Source: CAD feature listing. Evaluate the final solid. Frame: model axes, mm. A direction names the side the tool comes from. Round coordinates to 2 decimals unless told otherwise and drop trailing zeros. Order: outer loops, then holes, each group sorted by start corner. A loop starts at its lowest first (then second) coordinate and runs counter-clockwise, first axis right, second up. Notation, with made-up numbers: (46, 61.25) -> (64, 61.25) arc R26 ccw to (64, 80.25) -> close; hole circle Ø4 at (36.5, 33.5). An arc over 180 degrees is marked (long way). Write item = value, one per line. Start each with the question number.
(1) Cut plane A-A on y = -45. Return the cut outline in (x, z), then the cut area to 3 significant figures.
(2) Ray query, line 1 (Y direction, x = -73.5, z = 3.75); line 2 (X direction, y = -43.5, z = 10.5). Return the intervals inside material, ascending.
(3) Reachability of faces 1 (the face through (-82.914, -19, 9)), 2 (the face through (-63.864, -47, 9)) from +Z, -Z, +X, -X, +Y, -Y: full face, straight path, thin tool, end or side. Return the list, or none.
(4) Cut plane B-B on z = 16.75. Return the cut outline in (x, y), then the cut area to 3 significant figures.
(5) Contact query for flat-ended pins moving along their axis: pin 1 Ø5.5 at (y, z) = (-49.5, 10) entering from -X; pin 2 Ø10 at (x, z) = (-61, 6.5) entering from +Y; pin 3 Ø1 at (x, z) = (-72, 2.5) entering from -Y. Output: stop coordinate, or through.
(6) Cut plane C-C on x = -68. Return the cut outline in (y, z).
from build123d import *

# Parameters (mm, degrees)
F0_W     = 19.05
F0_H     = 19.05
F1_DEPTH = 38.1
F2_DEPTH = 57.15


with BuildPart() as f1:
    # F0 (on Front) → F1 (new body)
    with BuildSketch(Plane.XZ):
        with Locations((-73.389372, 9.525)):
            Rectangle(F0_W, F0_H)
    extrude(amount=F1_DEPTH)

    # F0 (on Front) → F2 (join)
    with BuildSketch(Plane.XZ):
        with Locations((-54.339372, 9.525)):
            Rectangle(F0_W, F0_H)
    extrude(amount=F2_DEPTH)


solid = f1.part
Evaluation:
q1.outline = (-63.86, 0) -> (-44.81, 0) -> (-44.81, 19.05) -> (-63.86, 19.05) -> close
q1.area = 363 mm^2
q2.line_1 = -38.1 to 0
q2.line_2 = -63.86 to -44.81
q3.face_1 = +Z, -Z, -X, +Y, -Y
q3.face_2 = +Z, -Z, -X, -Y
q4.outline = (-82.91, -38.1) -> (-63.86, -38.1) -> (-63.86, -57.15) -> (-44.81, -57.15) -> (-44.81, 0) -> (-82.91, 0) -> close
q4.area = 1,810 mm^2
q5.pin_1 = -63.86
q5.pin_2 = 0
q5.pin_3 = -38.1
q6.outline = (-38.1, 0) -> (0, 0) -> (0, 19.05) -> (-38.1, 19.05) -> close
